```python
from build123d import *

# Parameters (mm, degrees)
SKETCH1_W           = 700
SKETCH1_H           = 400
BOSS_EXTRUDE1_DEPTH = 40
FILLET1_R           = 10
SKETCH2_W           = 450
SKETCH2_H           = 200
BOSS_EXTRUDE2_DEPTH = 60
FILLET2_RADIUS      = 100
FILLET2_LENGTH      = 60
FILLET3_RADIUS      = 100
FILLET3_LENGTH      = 60


with BuildPart() as part:
    # Sketch1 → Boss-Extrude1 (new body)
    with BuildSketch(Plane(origin=(0, 0, 0), x_dir=(1, 0, 0), z_dir=(0, 1, 0))):
        Rectangle(SKETCH1_W, SKETCH1_H)
    extrude(amount=BOSS_EXTRUDE1_DEPTH)

    # Fillet1
    fillet1_edges = [part.edges().sort_by_distance(p)[0] for p in [
        (-350, 40, 0),
        (0, 40, 200),
        (350, 40, 0),
        (0, 0, 200),
        (-350, 0, 0),
        (0, 0, -200),
        (350, 0, 0),
        (350, 20, 200),
        (-350, 20, 200),
        (-350, 20, -200),
        (350, 20, -200),
        (0, 40, -200),
    ]]
    fillet(fillet1_edges, radius=FILLET1_R)

    # Sketch2 → Boss-Extrude2 (add)
    with BuildSketch(Plane(origin=(0, 40, 0), x_dir=(1, 0, 0), z_dir=(0, 1, 0))):
        Rectangle(SKETCH2_W, SKETCH2_H)
    extrude(amount=BOSS_EXTRUDE2_DEPTH)

    # Fillet2: full round fillet: the end face becomes a half cylinder, R = half its width
    fillet2_face = Plane((225, 70, 0), x_dir=(0, -1, 0), z_dir=(1, 0, 0))  # on the end face: x along it, z out of the body
    fillet2_slab = fillet2_face.offset(-FILLET2_RADIUS / 2) * Box(FILLET2_LENGTH, 2 * FILLET2_RADIUS, FILLET2_RADIUS, mode=Mode.PRIVATE)  # the body's end, R deep
    fillet2_round = Plane((125, 70, 0), x_dir=(1, 0, 0), z_dir=(0, -1, 0)) * Cylinder(FILLET2_RADIUS, FILLET2_LENGTH, mode=Mode.PRIVATE)  # its axis R under the face
    add(fillet2_slab - fillet2_round, mode=Mode.SUBTRACT)

    # Fillet3: full round fillet: the end face becomes a half cylinder, R = half its width
    fillet3_face = Plane((-225, 70, 0), x_dir=(0, -1, 0), z_dir=(-1, 0, 0))  # on the end face: x along it, z out of the body
    fillet3_slab = fillet3_face.offset(-FILLET3_RADIUS / 2) * Box(FILLET3_LENGTH, 2 * FILLET3_RADIUS, FILLET3_RADIUS, mode=Mode.PRIVATE)  # the body's end, R deep
    fillet3_round = Plane((-125, 70, 0), x_dir=(-1, 0, 0), z_dir=(0, -1, 0)) * Cylinder(FILLET3_RADIUS, FILLET3_LENGTH, mode=Mode.PRIVATE)  # its axis R under the face
    add(fillet3_slab - fillet3_round, mode=Mode.SUBTRACT)


solid = part.part
```
Read the model definition and answer for the solid it produces. Units are mm, in the model's axes. A direction names the side the tool comes from. Round coordinates to 2 decimals unless told otherwise and drop trailing zeros. Write each loop counter-clockwise with the first axis right and the second up, starting at its lowest first coordinate (ties: lowest second). Pieces come first, ordered by that corner, then holes. Notation, with made-up numbers: (-40, 54.25) - (-15, 54.25) arc R20 ccw to (-15, 74.25) - close; hole circle Ø10 at (10, 50). An arc over 180 degrees is marked (long way). Use CSV: the item, a comma, the result in double quotes.
Q1. Find section D-D, the plane z = 133.5. Write down the section's boundary in (x, y).
Values:
outline,"(-350, 10) arc R10 ccw to (-340, 0) - (340, 0) arc R10 ccw to (350, 10) - (350, 30) arc R10 ccw to (340, 40) - (-340, 40) arc R10 ccw to (-350, 30) - close"
Q2. Each of these flat-tipped pins is pushed along its axis until it touches: pin 1 Ø1 at (y, z) = (74, -40.5) entering from +X; pin 2 Ø8 at (y, z) = (42, 109) entering from -X; pin 3 Ø3 at (y, z) = (36.5, -23.5) entering from -X. Where does it stop, or does it pass through?
Values:
pin 1,"stops at x = 216.65"
pin 2,"stops at x = -346"
pin 3,"stops at x = -348.66"
Q3. Find section A-A, the plane x = -100. Write down the section's boundary in (y, z).
Values:
outline,"(0, -190) arc R10 ccw to (10, -200) - (30, -200) arc R10 ccw to (40, -190) - (40, -100) - (100, -100) - (100, 100) - (40, 100) - (40, 190) arc R10 ccw to (30, 200) - (10, 200) arc R10 ccw to (0, 190) - close"
Q4. Find section C-C, the plane y = 79. Write down the section's boundary in (x, z).
Values:
outline,"(-125, -100) - (125, -100) arc R100 ccw to (125, 100) - (-125, 100) arc R100 ccw to start"
Q5. A tool of negligible diameter and unlimited length cuts with its end or side. For faces 1 (the cylindrical face through (-224.976, 69.58, 2.199)), 2 (the flat face through (-5, 40, -129)), 3 (the cylindrical face through (224.976, 69.58, -2.199)), 4 (the flat face through (-2, 70, -100)), 5 (the flat face through (-2, 70, 100)), from which of +Z, -Z, +X, -X, +Y, -Y can it reach the whole face along a straight path? Write none if from no direction.
Values:
face 1,"-X, +Y"
face 2,"+Y"
face 3,"+X, +Y"
face 4,"-Z, +X, -X, +Y"
face 5,"+Z, +X, -X, +Y"
Q6. Straight lines are drawn through the part: line 1 along X through (y, z) = (70, 66); line 2 along Z through (x, y) = (37.5, 54); line 3 along Y through (x, z) = (-95, -182). For each, find the intervals that lie inside material, in ascending order.
Values:
line 1,"x = -200.13 to 200.13"
line 2,"z = -100 to 100"
line 3,"y = 0 to 40"
Q7. Find section B-B, the plane z = -46.5. Write down the section's boundary in (x, y), then the cut area to 3 significant figures.
Values:
outline,"(-350, 10) arc R10 ccw to (-340, 0) - (340, 0) arc R10 ccw to (350, 10) - (350, 30) arc R10 ccw to (340, 40) - (213.53, 40) - (213.53, 100) - (-213.53, 100) - (-213.53, 40) - (-340, 40) arc R10 ccw to (-350, 30) - close"
area,"53,500 mm²"
